Autodesk Inventor part; units mm, degrees
ref_plane "YZ Plane" through (0, 0, 0) normal (1, 0, 0) x (0, 1, 0)
ref_plane "XZ Plane" through (0, 0, 0) normal (0, 1, 0) x (-1, 0, 0)
ref_plane "XY Plane" through (0, 0, 0) normal (0, 0, 1) x (1, 0, 0)
sketch "Esboço2" plane through (0, 0, 0) normal (0, 1, 0) x (-1, 0, 0)
  circle A0 centre (0, 0) radius 1.5
  line L0 (2.7, -1.5588) -> (0, -3.1177)
  line L1 (0, -3.1177) -> (-2.7, -1.5588)
  line L2 (-2.7, -1.5588) -> (-2.7, 1.5588)
  line L3 (-2.7, 1.5588) -> (0, 3.1177)
  line L4 (0, 3.1177) -> (2.7, 1.5588)
  line L5 (2.7, 1.5588) -> (2.7, -1.5588)
extrude "Extrusão1" add sketch "Esboço2" along normal blind 2.4
thread "Rosca1"
chamfer "Chanfro1" distance 0.3 angle 45 2 edges at (1.5, 2.4, 0) (1.5, 0, 0)
sketch "Esboço3" plane through (0, 0, 0) normal (0, 0, 1) x (1, 0, 0)
  line L0 (0, -0.6576) -> (0, 3.9457)
  line L1 (2.4, 2.4) -> (4.5158, 1.4134)
  line L2 (2.4, 2.4) -> (4.7345, 2.4) construction
  line L3 (2.4, 0) -> (4.5158, 0.9866)
  line L4 (2.4, 2.4) -> (4.5158, 2.4)
  line L5 (2.4, 0) -> (4.5158, 0.9866)
  line L6 (2.4, 2.4) -> (4.5158, 1.4134)
  line L7 (4.5158, 1.4134) -> (4.5158, 2.4)
  line L8 (4.5158, 0.9866) -> (4.5158, 0)
  line L9 (4.5158, 0.9866) -> (2.4, 0)
  line L10 (2.4, 0) -> (4.5158, 0)
  line L11 (2.7, 0) -> (0, 0)
  dimension "d16" = 25
revolve "Revolução2" cut sketch "Esboço3" angle 360 about axis through (0, -10, 0) along (0, 1, 0)
properties part number "porca m3" material "Aço galvanizado"
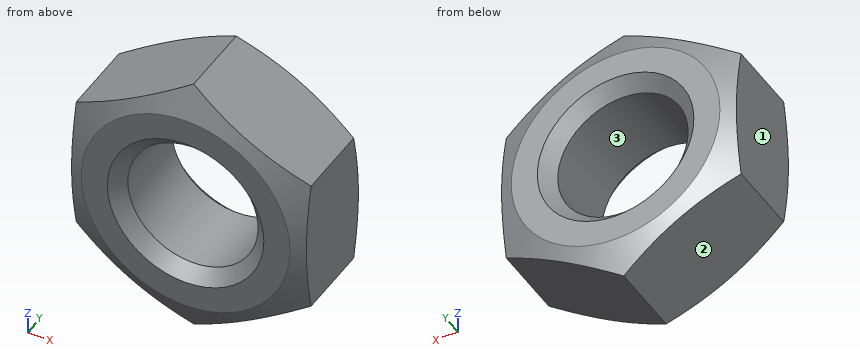
The listing builds one solid part. Answer for the finished solid, in the listing's coordinates (mm). Face numbers are marked on the shaded views. Coordinates: 2 decimals unless noted, no trailing zeros. Write each loop counter-clockwise with the first axis right and the second up, starting at its lowest first coordinate (ties: lowest second). Pieces come first, ordered by that corner, then holes. Notation, with made-up numbers: M 47.25,10 L 60.25,10 A28 cw 60.25,41 Z; hole C -33,81 d11. An arc over 180 degrees is marked long. Use a Markdown table: item, result. Add a question column.
1. For a pull along Z with two mould halves and no side action, classify the marked faces 1, 2 and 3 as +Z half, -Z half, draft (parallel to the pull), parting line (faces both ways), or undercut.
2. Straight lines are drawn through the part: line 1 along X through (y, z) = (1.7, 0.25); line 2 along Z through (x, y) = (-1.2, 0.2); line 3 along Z through (x, y) = (0.8, 0.35). For each, find the intervals that lie inside material, in ascending order. Write a range as [from, to].
3. Section A-A (y = 1) is taken. Give the vertices of the cut face in (x, z).
4. Given P1, Ø1, axis at x = 2, z = -1.5, coming from the +Y side, flat-ended and moving along its own axis, determine where the tip first touches the part or whether it passes through.
5. Section B-B (z = 0) is taken. Give the vertices of the cut face in (x, y), plus the area to 3 significant figures.
Data:
| question | item | result |
|---|---|---|
| 1 | face 1 | draft |
| 1 | face 2 | -Z half |
| 1 | face 3 | undercut |
| 2 | line 1 | x = [-2.7, -1.48], [1.48, 2.7] |
| 2 | line 2 | z = [-2.42, -1.06], [1.06, 2.42] |
| 2 | line 3 | z = [-2.66, -1.27], [1.27, 2.66] |
| 3 | outline | M -2.7,-1.56 L 0,-3.12 L 2.7,-1.56 L 2.7,1.56 L 0,3.12 L -2.7,1.56 Z; hole C 0,0 d3 |
| 4 | P1 | stops at y = 2.4 |
| 5 | outline | M -2.7,0.14 L -2.4,0 L -1.8,0 L -1.5,0.3 L -1.5,2.1 L -1.8,2.4 L -2.4,2.4 L -2.7,2.26 Z; M 1.5,0.3 L 1.8,0 L 2.4,0 L 2.7,0.14 L 2.7,2.26 L 2.4,2.4 L 1.8,2.4 L 1.5,2.1 Z |
| 5 | area | 5.50 mm2 |
